Geometry: final body of the model. Coordinates: model frame, mm. Give positions to 0.01 mm unless a question says otherwise; leave off trailing zeros. Loops run counter-clockwise (first coordinate to the right, second up) from the corner with the lowest first, then second, coordinate; pieces in that order, holes last.
1. First-contact query: P1, Ø5, axis at y = -15.07, z = -53.85, coming from the +X side; P2, Ø1.5, axis at x = 2, y = 20.5, coming from the -Z side; P3, Ø1.5, axis at x = 0.5, y = -11.5, coming from the -Z side; P4, Ø1.5, axis at x = 1, z = -36.5, coming from the +Y side. Flat tips, straight axial feed; report the tip coordinate or a pass-through.
2. Section C-C, the plane y = 16.5. Output: boundary loops of the cut face in (x, z), then the cut area to 3 significant figures.
3. Material intervals for line 1 along Y through (x, z) = (2.8, -30.5); line 2 along Z through (x, y) = (0.5, 16); line 3 along Y through (x, z) = (0.9, -1), sorted ascending.
4. Section D-D, the plane x = 1.05. State how many separate pieces and enclosed holes the cut face has, then the cut area to 3 significant figures.
5. Section A-A, the plane y = -3. Output: boundary loops of the cut face in (x, z).
6. Section B-B, the plane z = -27.5. Output: boundary loops of the cut face in (x, y), then the cut area to 3 significant figures.
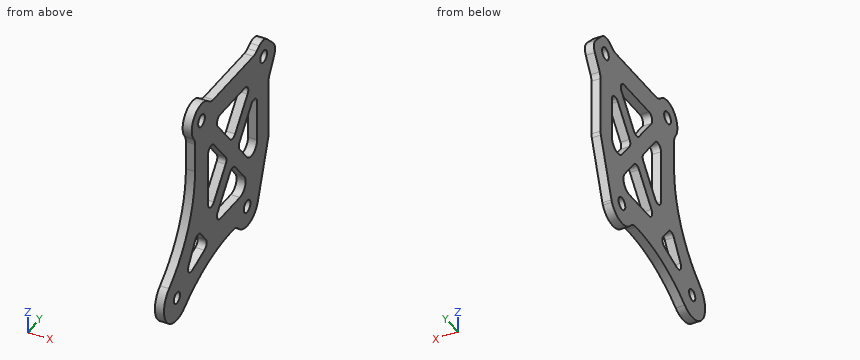
from build123d import *

# Parameters (mm, degrees)
SKETCH_1_R          = 1.9
SKETCH_1_R_2        = 2.05
EXTRUDE_1_DEPTH     = 3
EXTRUDE_2_DEPTH     = 3
CUT_EXTRUDE_1_DEPTH = 10
FILLET_1_R          = 2
FILLET_2_R          = 4
FILLET_3_R          = 3.5
CUT_EXTRUDE_2_DEPTH = 10
FILLET_4_R          = 2


with BuildPart() as part:
    # 草图1 → 凸台-拉伸1 (new body)
    with BuildSketch(Plane(origin=(0, 0, 0), x_dir=(0, 0, -1), z_dir=(1, 0, 0))):
        with BuildLine():
            Line((-3, 40.986839826), (-3, 5.196152423))
            ThreePointArc((-3, 5.196152423), (-4.656619043, -3.783635697), (4.472135955, -4))
            Line((4.472135955, -4), (15.668888745, -4))
            ThreePointArc((15.668888745, -4), (33.469294357, -8.178978797), (47.550324088, -19.842721997))
            ThreePointArc((47.550324088, -19.842721997), (58.506158977, -21.45142262), (60.307864912, -10.525669029))
            ThreePointArc((60.307864912, -10.525669029), (53.0476279, 4.779832589), (51.314694229, 21.631134085))
            ThreePointArc((51.314694229, 21.631134085), (55.199709707, 27.963749659), (51.2, 34.22455532))
            Line((51.2, 34.22455532), (51.2, 40.986839826))
            Line((51.2, 40.986839826), (-3, 40.986839826))
        make_face()
        with Locations((53.846907568, -15.071659592)):
            Circle(SKETCH_1_R, mode=Mode.SUBTRACT)
        Circle(SKETCH_1_R_2, mode=Mode.SUBTRACT)
        Polygon((5, 7.211107417), (5, 30.775732409), (19.616479342, 18.993419913), align=None, mode=Mode.SUBTRACT)
        Polygon((38.216479342, 4), (8.983520658, 4), (23.6, 15.782312496), align=None, mode=Mode.SUBTRACT)
        with Locations((1, 37.986839826)):
            Circle(SKETCH_1_R_2, mode=Mode.SUBTRACT)
        Polygon((8.983520658, 33.986839826), (38.216479342, 33.986839826), (23.6, 22.204527331), align=None, mode=Mode.SUBTRACT)
        Polygon((27.583520658, 18.993419913), (42.2, 30.775732409), (42.2, 7.211107417), align=None, mode=Mode.SUBTRACT)
        with Locations((48.2, 27.9)):
            Circle(SKETCH_1_R_2, mode=Mode.SUBTRACT)
    extrude(amount=EXTRUDE_1_DEPTH)

    # 草图2 → 凸台-拉伸2 (add)
    with BuildSketch(Plane(origin=(3, 0, 0), x_dir=(0, 0, -1), z_dir=(1, 0, 0))):
        Polygon((10.660254038, 40.986839826), (2, 45.986839826), (-3, 40.986839826), align=None)
        Polygon((-3, 32.790687404), (-3, 40.986839826), (-6, 37.986839826), align=None)
    extrude(amount=-EXTRUDE_2_DEPTH)

    # 草图3 → 切除-拉伸1 (cut)
    with BuildSketch(Plane(origin=(3, 0, 0), x_dir=(0, 0, -1), z_dir=(1, 0, 0))):
        Polygon((51.2, 34.22455532), (31.2, 40.986839826), (51.2, 40.986839826), align=None)
    extrude(amount=-CUT_EXTRUDE_1_DEPTH, mode=Mode.SUBTRACT)

    # 圆角1
    fillet_1_edges = [part.edges().sort_by_distance(p)[0] for p in [
        (1.5, 22.204527331, -23.6),
        (1.5, 33.986839826, -8.983520658),
        (1.5, 30.775732409, -5),
        (1.5, 7.211107417, -5),
        (1.5, 18.993419913, -19.616479342),
        (1.5, 7.211107417, -42.2),
        (1.5, 18.993419913, -27.583520658),
        (1.5, 4, -8.983520658),
        (1.5, 4, -38.216479342),
        (1.5, 15.782312496, -23.6),
    ]]
    fillet(fillet_1_edges, radius=FILLET_1_R)

    # 圆角2
    fillet_2_edges = [part.edges().sort_by_distance(p)[0] for p in [
        (1.5, -4, -4.472135955),
        (1.5, 5.196152423, 3),
        (1.5, 34.22455532, -51.2),
        (1.5, 21.631134085, -51.314694229),
        (1.5, 45.986839826, -2),
        (1.5, 40.986839826, -10.660254038),
        (1.5, 37.986839826, 6),
        (1.5, 32.790687404, 3),
        (1.5, 40.986839826, -31.2),
    ]]
    fillet(fillet_2_edges, radius=FILLET_2_R)

    # 圆角3
    fillet_3_edges = [part.edges().sort_by_distance(p)[0] for p in [
        (1.5, 33.986839826, -38.216479342),
        (1.5, 30.775732409, -42.2),
    ]]
    fillet(fillet_3_edges, radius=FILLET_3_R)

    # 草图4 → 切除-拉伸2 (cut)
    with BuildSketch(Plane(origin=(3, 0, 0), x_dir=(0, 0, -1), z_dir=(1, 0, 0))):
        Polygon((37.863150267, -2.349540483), (46.512425203, 4.497802174), (51.661041238, -10.892084105), align=None)
    extrude(amount=-CUT_EXTRUDE_2_DEPTH, mode=Mode.SUBTRACT)

    # 圆角4
    fillet_4_edges = [part.edges().sort_by_distance(p)[0] for p in [
        (1.5, -10.892084105, -51.661041238),
        (1.5, -2.349540483, -37.863150267),
        (1.5, 4.497802174, -46.512425203),
    ]]
    fillet(fillet_4_edges, radius=FILLET_4_R)


solid = part.part
Answers below:
1. P1: stops at x = 3
1. P2: stops at z = -51.65
1. P3: stops at z = -61.23
1. P4: stops at y = 39.45
2. outline: (0, -51.23) - (3, -51.23) - (3, -42.2) - (0, -42.2) - close; (0, -30.68) - (3, -30.68) - (3, -16.52) - (0, -16.52) - close; (0, -5) - (3, -5) - (3, 3) - (0, 3) - close
2. area: 93.6 mm2
3. line 1: y = -6.85 to 4, 10.22 to 16.64, 21.34 to 27.77, 33.21 to 40.99
3. line 2: z = -51.25 to -42.2, -31.3 to -15.9, -5 to 3
3. line 3: y = -5.92 to -1.79, 1.79 to 35.94, 40.04 to 44.63
4. separate pieces: 1
4. enclosed holes: 9
4. area: 2,150 mm2
5. outline: (0, -55.94) - (3, -55.94) - (3, -49.02) - (0, -49.02) - close; (0, -39.53) - (3, -39.53) - (3, 5.2) - (0, 5.2) - close
6. outline: (0, -5.79) - (3, -5.79) - (3, 4) - (0, 4) - close; (0, 12.64) - (3, 12.64) - (3, 25.35) - (0, 25.35) - close; (0, 33.99) - (3, 33.99) - (3, 40.99) - (0, 40.99) - close
6. area: 88.5 mm2
